Part model, mm, in its own coordinate system. Face numbers are marked on the shaded views. A direction names the side the tool comes from. Round coordinates to 2 decimals unless told otherwise and drop trailing zeros. Write each loop counter-clockwise with the first axis right and the second up, starting at its lowest first coordinate (ties: lowest second). Pieces come first, ordered by that corner, then holes.
from build123d import *

# Parameters (mm, degrees)
SKETCH1_W            = 300
SKETCH1_H            = 20
BOSS_EXTRUDE1_DEPTH  = 8
SKETCH2_W            = 34
SKETCH2_H            = 8
BOSS_EXTRUDE2_DEPTH  = 9
SKETCH3_W            = 34
SKETCH3_H            = 8
BOSS_EXTRUDE3_DEPTH  = 9
SKETCH4_R            = 1.45
CUT_EXTRUDE1_DEPTH   = 302.504560496
SKETCH5_W            = 25
SKETCH5_H            = 8
BOSS_EXTRUDE4_DEPTH  = 17
SKETCH6_W            = 25
SKETCH6_H            = 8
BOSS_EXTRUDE5_DEPTH  = 17
SKETCH7_W            = 10
SKETCH7_H            = 38
CUT_EXTRUDE2_DEPTH   = 303.37890138
SKETCH8_W            = 7
SKETCH8_H            = 16
CUT_EXTRUDE3_DEPTH   = 4
CUT_EXTRUDE4_DEPTH   = 7
BOSS_EXTRUDE6_DEPTH  = 10
SKETCH12_W           = 8
SKETCH12_H           = 8
BOSS_EXTRUDE7_DEPTH  = 17
SKETCH13_R           = 1.7
CUT_EXTRUDE6_DEPTH   = 305.926220585
SKETCH14_W           = 20
SKETCH14_H           = 13
BOSS_EXTRUDE8_DEPTH  = 12
SKETCH15_R           = 1.6
CUT_EXTRUDE7_DEPTH   = 20
SKETCH16_W           = 20
SKETCH16_H           = 13
BOSS_EXTRUDE9_DEPTH  = 12
SKETCH17_R           = 1.6
CUT_EXTRUDE8_DEPTH   = 20
SKETCH18_W           = 20
SKETCH18_H           = 13
BOSS_EXTRUDE10_DEPTH = 12
CUT_EXTRUDE9_START   = -20
SKETCH19_R           = 1.6
CUT_EXTRUDE9_DEPTH   = 20
SKETCH20_W           = 20
SKETCH20_H           = 13
BOSS_EXTRUDE11_DEPTH = 12
CUT_EXTRUDE10_START  = -20
SKETCH21_R           = 1.6
CUT_EXTRUDE10_DEPTH  = 20
FILLET6_R            = 3
SKETCH22_W           = 123.750788161
SKETCH22_H           = 72.639217631
CUT_EXTRUDE11_DEPTH  = 244
SKETCH23_R           = 1.6
CUT_EXTRUDE12_DEPTH  = 71.611613776
FILLET7_R            = 3
SKETCH24_W           = 5.5
SKETCH24_H           = 78.243551934
CUT_EXTRUDE13_DEPTH  = 0.8
SKETCH25_W           = 20
SKETCH25_H           = 5.75655834
CUT_EXTRUDE14_DEPTH  = 0.5
SKETCH26_W           = 20
SKETCH26_H           = 21.459079842
CUT_EXTRUDE15_DEPTH  = 0.5


with BuildPart() as part:
    # Sketch1 → Boss-Extrude1 (new body)
    with BuildSketch(Plane(origin=(0, 0, 0), x_dir=(1, 0, 0), z_dir=(0, 1, 0))):
        with Locations((150, -10)):
            Rectangle(SKETCH1_W, SKETCH1_H)
    extrude(amount=BOSS_EXTRUDE1_DEPTH)

    # Sketch2 → Boss-Extrude2 (add)
    with BuildSketch(Plane.XY.offset(20)):
        with Locations((17, 4)):
            Rectangle(SKETCH2_W, SKETCH2_H)
        with Locations((283, 4)):
            Rectangle(SKETCH2_W, SKETCH2_H)
    extrude(amount=BOSS_EXTRUDE2_DEPTH)

    # Sketch3 → Boss-Extrude3 (add)
    with BuildSketch(Plane(origin=(0, 0, 0), x_dir=(-1, 0, 0), z_dir=(0, 0, -1))):
        with Locations((-17, 4)):
            Rectangle(SKETCH3_W, SKETCH3_H)
        with Locations((-283, 4)):
            Rectangle(SKETCH3_W, SKETCH3_H)
    extrude(amount=BOSS_EXTRUDE3_DEPTH)

    # Sketch4 → Cut-Extrude1 (cut, through all)
    with BuildSketch(Plane(origin=(0, 8, 0), x_dir=(1, 0, 0), z_dir=(0, 1, 0))):
        with Locations(Location((4, 5, 0), (0, 0, 270))):
            Circle(SKETCH4_R)
        with Locations(Location((30, 5, 0), (0, 0, 270))):
            Circle(SKETCH4_R)
        with Locations(Location((30, -25, 0), (0, 0, 270))):
            Circle(SKETCH4_R)
        with Locations(Location((4, -25, 0), (0, 0, 270))):
            Circle(SKETCH4_R)
        with Locations(Location((296, -25, 0), (0, 0, 270))):
            Circle(SKETCH4_R)
        with Locations(Location((296, 5, 0), (0, 0, 270))):
            Circle(SKETCH4_R)
        with Locations(Location((270, -25, 0), (0, 0, 270))):
            Circle(SKETCH4_R)
        with Locations(Location((270, 5, 0), (0, 0, 270))):
            Circle(SKETCH4_R)
    extrude(amount=-CUT_EXTRUDE1_DEPTH, mode=Mode.SUBTRACT)

    # Sketch5 → Boss-Extrude4 (add)
    with BuildSketch(Plane.XY.offset(20)):
        with Locations((253.5, 4)):
            Rectangle(SKETCH5_W, SKETCH5_H)
    extrude(amount=BOSS_EXTRUDE4_DEPTH)

    # Sketch6 → Boss-Extrude5 (add)
    with BuildSketch(Plane(origin=(0, 0, 0), x_dir=(-1, 0, 0), z_dir=(0, 0, -1))):
        with Locations((-253.5, 4)):
            Rectangle(SKETCH6_W, SKETCH6_H)
    extrude(amount=BOSS_EXTRUDE5_DEPTH)

    # Sketch7 → Cut-Extrude2 (cut, through all)
    with BuildSketch(Plane(origin=(0, 8, 0), x_dir=(1, 0, 0), z_dir=(0, 1, 0))):
        with Locations((254, -10)):
            Rectangle(SKETCH7_W, SKETCH7_H)
    extrude(amount=-CUT_EXTRUDE2_DEPTH, mode=Mode.SUBTRACT)

    # Sketch8 → Cut-Extrude3 (cut)
    with BuildSketch(Plane(origin=(0, 8, 0), x_dir=(1, 0, 0), z_dir=(0, 1, 0))):
        with Locations((262.5, -10)):
            Rectangle(SKETCH8_W, SKETCH8_H)
    extrude(amount=-CUT_EXTRUDE3_DEPTH, mode=Mode.SUBTRACT)

    # Sketch9 → Cut-Extrude4 (cut)
    with BuildSketch(Plane.ZY.offset(-259)):
        Polygon((18, 4), (22, 8), (18, 8), align=None)
        Polygon((2, 4), (-2, 8), (2, 8), align=None)
    extrude(amount=-CUT_EXTRUDE4_DEPTH, mode=Mode.SUBTRACT)

    # Sketch10 → Boss-Extrude6 (add)
    with BuildSketch(Plane.ZY.offset(-259)):
        Polygon((-2, 0), (-9, 8), (-9, 0), align=None)
        Polygon((29, 8), (22, 0), (29, 0), align=None)
    extrude(amount=BOSS_EXTRUDE6_DEPTH)

    # Sketch12 → Boss-Extrude7 (add)
    with BuildSketch(Plane.XY.offset(37)):
        with Locations((245, 4)):
            Rectangle(SKETCH12_W, SKETCH12_H)
    extrude(amount=BOSS_EXTRUDE7_DEPTH)

    # Sketch13 → Cut-Extrude6 (cut, through all)
    with BuildSketch(Plane(origin=(0, 8, 0), x_dir=(1, 0, 0), z_dir=(0, 1, 0))):
        with Locations(Location((245, -50, 0), (0, 0, 270))):
            Circle(SKETCH13_R)
        with Locations(Location((245, -18, 0), (0, 0, 270))):
            Circle(SKETCH13_R)
    extrude(amount=-CUT_EXTRUDE6_DEPTH, mode=Mode.SUBTRACT)

    # Sketch14 → Boss-Extrude8 (add)
    with BuildSketch(Plane.XY.offset(29)):
        with Locations((285, 6.5)):
            Rectangle(SKETCH14_W, SKETCH14_H)
    extrude(amount=BOSS_EXTRUDE8_DEPTH)

    # Sketch15 → Cut-Extrude7 (cut)
    with BuildSketch(Plane(origin=(295, 0, 0), x_dir=(0, 0, -1), z_dir=(1, 0, 0))):
        with Locations((-35, 8)):
            Circle(SKETCH15_R)
    extrude(amount=-CUT_EXTRUDE7_DEPTH, mode=Mode.SUBTRACT)

    # Sketch16 → Boss-Extrude9 (add)
    with BuildSketch(Plane(origin=(0, 0, -9), x_dir=(-1, 0, 0), z_dir=(0, 0, -1))):
        with Locations((-285, 6.5)):
            Rectangle(SKETCH16_W, SKETCH16_H)
    extrude(amount=BOSS_EXTRUDE9_DEPTH)

    # Sketch17 → Cut-Extrude8 (cut)
    with BuildSketch(Plane(origin=(295, 0, 0), x_dir=(0, 0, -1), z_dir=(1, 0, 0))):
        with Locations((15, 8)):
            Circle(SKETCH17_R)
    extrude(amount=-CUT_EXTRUDE8_DEPTH, mode=Mode.SUBTRACT)

    # Sketch18 → Boss-Extrude10 (add)
    with BuildSketch(Plane(origin=(0, 0, -9), x_dir=(-1, 0, 0), z_dir=(0, 0, -1))):
        with Locations((-15, 6.5)):
            Rectangle(SKETCH18_W, SKETCH18_H)
    extrude(amount=BOSS_EXTRUDE10_DEPTH)

    # Sketch19 → Cut-Extrude9 (cut)
    with BuildSketch(Plane.ZY.offset(-5).offset(CUT_EXTRUDE9_START)):
        with Locations(Location((-15, 8, 0), (0, 0, 180))):
            Circle(SKETCH19_R)
    extrude(amount=CUT_EXTRUDE9_DEPTH, mode=Mode.SUBTRACT)

    # Sketch20 → Boss-Extrude11 (add)
    with BuildSketch(Plane.XY.offset(29)):
        with Locations((15, 6.5)):
            Rectangle(SKETCH20_W, SKETCH20_H)
    extrude(amount=BOSS_EXTRUDE11_DEPTH)

    # Sketch21 → Cut-Extrude10 (cut)
    with BuildSketch(Plane.ZY.offset(-5).offset(CUT_EXTRUDE10_START)):
        with Locations(Location((35, 8, 0), (0, 0, 180))):
            Circle(SKETCH21_R)
    extrude(amount=CUT_EXTRUDE10_DEPTH, mode=Mode.SUBTRACT)

    # Fillet6
    fillet6_edges = [part.edges().sort_by_distance(p)[0] for p in [
        (285, 13, 29),
        (285, 13, 41),
        (285, 13, -9),
        (285, 13, -21),
        (15, 13, -9),
        (15, 13, -21),
        (15, 13, 29),
        (15, 13, 41),
    ]]
    fillet(fillet6_edges, radius=FILLET6_R)

    # Sketch22 → Cut-Extrude11 (cut)
    with BuildSketch(Plane(origin=(300, 0, 0), x_dir=(0, 0, -1), z_dir=(1, 0, 0))):
        with Locations((-10.128058827, -1.301866478)):
            Rectangle(SKETCH22_W, SKETCH22_H)
    extrude(amount=-CUT_EXTRUDE11_DEPTH, mode=Mode.SUBTRACT)

    # Sketch23 → Cut-Extrude12 (cut, through all)
    with BuildSketch(Plane(origin=(0, 0, 0), x_dir=(-1, 0, 0), z_dir=(0, -1, 0))):
        with Locations(Location((-51, -5, 0), (0, 0, 90))):
            Circle(SKETCH23_R)
        with Locations(Location((-51, -15, 0), (0, 0, 90))):
            Circle(SKETCH23_R)
        with Locations(Location((-43, -5, 0), (0, 0, 90))):
            Circle(SKETCH23_R)
        with Locations(Location((-43, -15, 0), (0, 0, 90))):
            Circle(SKETCH23_R)
    extrude(amount=-CUT_EXTRUDE12_DEPTH, mode=Mode.SUBTRACT)

    # Fillet7
    fillet7_edges = [part.edges().sort_by_distance(p)[0] for p in [
        (0, 4, 29),
        (34, 4, 29),
        (0, 4, -9),
        (34, 4, -9),
    ]]
    fillet(fillet7_edges, radius=FILLET7_R)

    # Sketch24 → Cut-Extrude13 (cut)
    with BuildSketch(Plane(origin=(0, 13, 0), x_dir=(1, 0, 0), z_dir=(0, 1, 0))):
        with Locations((15, -9.577024089)):
            Rectangle(SKETCH24_W, SKETCH24_H)
    extrude(amount=-CUT_EXTRUDE13_DEPTH, mode=Mode.SUBTRACT)

    # Sketch25 → Cut-Extrude14 (cut)
    with BuildSketch(Plane(origin=(0, 0, 29), x_dir=(-1, 0, 0), z_dir=(0, 0, -1))):
        with Locations((-15, 10.87827917)):
            Rectangle(SKETCH25_W, SKETCH25_H)
    extrude(amount=-CUT_EXTRUDE14_DEPTH, mode=Mode.SUBTRACT)

    # Sketch26 → Cut-Extrude15 (cut)
    with BuildSketch(Plane.XY.offset(-9)):
        with Locations((15, 18.729539921)):
            Rectangle(SKETCH26_W, SKETCH26_H)
    extrude(amount=-CUT_EXTRUDE15_DEPTH, mode=Mode.SUBTRACT)


solid = part.part
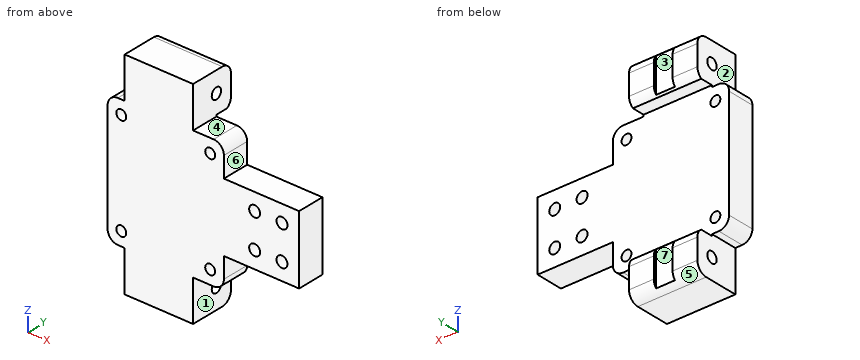
Q1. Saw through at C-C, the plane x = 43. Write the cut outline in (y, z).
Q2. Drop flat-ended pins along their axis: P1, Ø5, axis at x = 50, z = 6, coming from the +Y side; P2, Ø3, axis at x = 14.5, z = 28.5, coming from the +Y side; P3, Ø1.5, axis at y = 8, z = 33.5, coming from the +X side. Give the stop position or say it passes through.
Q3. Two-plate mould, pull along X, no slides. Class the marked faces 5, 6 and 7: released by +X, released by -X, zero draft, split by the parting line, or undercut.
Q4. Saw through at B-B, the plane z = -15. Write the cut outline in (x, y).
Q5. Wall check: line 1 (X direction, y = 3.5, z = 15); line 2 (X direction, y = 4, z = 25); line 3 (Y direction, x = 14.5, z = -15). Give the ranges that are in metal, low to high.
Q6. Saw through at D-D, the plane z = 15. Write the cut outline in (x, y), and give its area (3 significant figures).
Q7. Tool access for the marked faces 1, 2, 3 and 4: list every direction of +Z, -Z, +X, -X, +Y, -Y with a clear straight run to the whole face (end or side of a thin tool).
Q8. Saw through at A-A, the plane x = 15.5. Write the cut outline in (y, z), and give its area (3 significant figures).
Computed:
1. outline: (0, 0) - (8, 0) - (8, 3.4) - (0, 3.4) - close; (0, 6.6) - (8, 6.6) - (8, 13.4) - (0, 13.4) - close; (0, 16.6) - (8, 16.6) - (8, 20) - (0, 20) - close
2. P1: stops at y = 8
2. P2: stops at y = 12.2
2. P3: stops at x = 25
3. face 5: zero draft
3. face 6: released by +X
3. face 7: undercut
4. outline: (5, 0) - (25, 0) - (25, 6.4) - (5, 6.4) - close; (5, 9.6) - (25, 9.6) - (25, 13) - (17.75, 13) - (17.75, 12.2) - (12.25, 12.2) - (12.25, 13) - (5, 13) - close
5. line 1: x = 0 to 41.4, 44.6 to 49.4, 52.6 to 56
5. line 2: x = 0 to 2.55, 5.45 to 28.55, 31.45 to 34
5. line 3: y = 0 to 6.4, 9.6 to 12.2
6. outline: (0, 0) - (41.4, 0) - (41.4, 8) - (0, 8) - close; (44.6, 0) - (49.4, 0) - (49.4, 8) - (44.6, 8) - close; (52.6, 0) - (56, 0) - (56, 8) - (52.6, 8) - close
6. area: 397 mm2
7. face 1: -Z, +X, +Y, -Y
7. face 2: +Z, -X, +Y, -Y
7. face 3: +Z, -Z, +Y
7. face 4: +Z, +X, +Y, -Y
8. outline: (0, -21) - (10, -21) arc R3 ccw to (12.2, -20.04) - (12.2, -9.96) arc R3 ccw to (11.66, -9.5) - (8, -9.5) - (8, 29.5) - (11.66, 29.5) arc R3 ccw to (12.2, 29.96) - (12.2, 40.04) arc R3 ccw to (10, 41) - (0, 41) - close; hole circle Ø3.2 at (8, -15); hole circle Ø3.2 at (8, 35)
8. area: 575 mm2
